For this review, use the dimensioned drawing (mm, ordinates from the lowest corner) and the shaded views. Give positions to 0.01 mm unless a question says otherwise; leave off trailing zeros. Loops run counter-clockwise (first coordinate to the right, second up) from the corner with the lowest first, then second, coordinate; pieces in that order, holes last. Notation, with made-up numbers: (-5.75, -19) -> (53.25, -19) arc R15 ccw to (53.25, 6) -> close; hole circle Ø7 at (33.25, -31.5). An arc over 180 degrees is marked (long way). Write each question's results on one line, items separated by ' | '. Start each with the question number.
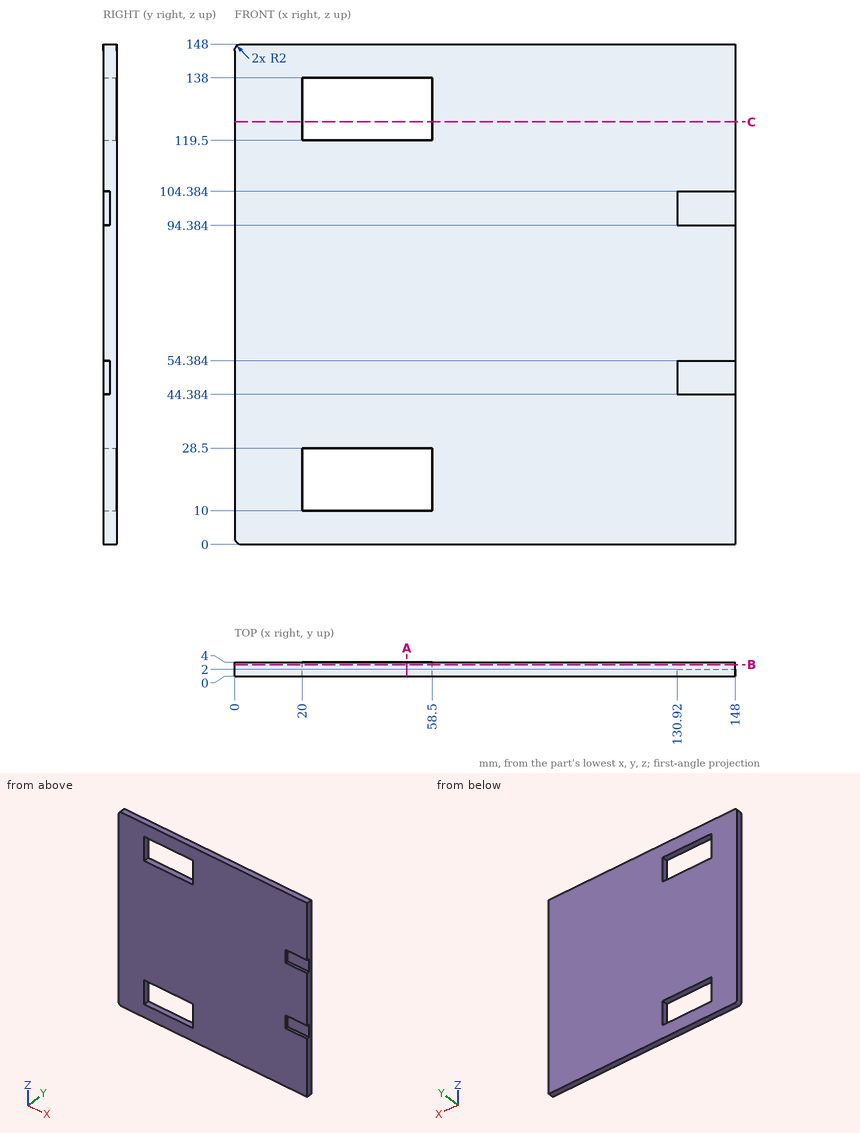
1. We need section C-C (z = 125). Write out the cut boundary in (x, y).
2. Wall thickness on L1, parallel to Z at x = 56, y = 0.6; L2, parallel to X at y = 3.3, z = 135.5; L3, parallel to X at y = 1.3, z = 45: over which ranges is each line inside the solid? List them lowest first.
3. For pin 1 Ø11 at (x, z) = (136.5, 99.5) entering from -Y; pin 2 Ø3 at (x, z) = (143.5, 47.5) entering from -Y, all flat-tipped, find the tip position at first contact; note any pin that passes through.
4. We need section A-A (x = 51). Write out the cut boundary in (y, z), plus the area to 3 significant figures.
5. We need section B-B (y = 3.4). Write out the cut boundary in (x, z), plus the area to 3 significant figures.
Response:
1) outline: (0, 0) -> (20, 0) -> (20, 4) -> (0, 4) -> close; (58.5, 0) -> (148, 0) -> (148, 4) -> (58.5, 4) -> close
2) L1: z = 0 to 10, 28.5 to 119.5, 138 to 148 | L2: x = 0 to 20, 58.5 to 148 | L3: x = 0 to 130.92
3) pin 1: stops at y = 0 | pin 2: stops at y = 2
4) outline: (0, 0) -> (4, 0) -> (4, 10) -> (0, 10) -> close; (0, 28.5) -> (4, 28.5) -> (4, 119.5) -> (0, 119.5) -> close; (0, 138) -> (4, 138) -> (4, 148) -> (0, 148) -> close | area: 444 mm2
5) outline: (0, 2) arc R2 ccw to (2, 0) -> (148, 0) -> (148, 148) -> (2, 148) arc R2 ccw to (0, 146) -> close; hole (20, 10) -> (58.5, 10) -> (58.5, 28.5) -> (20, 28.5) -> close; hole (20, 119.5) -> (58.5, 119.5) -> (58.5, 138) -> (20, 138) -> close | area: 20,500 mm2
